Verification items for this drawing (mm, ordinates from the low corner). A direction names the side the tool comes from. Coordinates: 2 decimals unless noted, no trailing zeros. Order: outer loops, then holes, each group sorted by start corner. A loop starts at its lowest first (then second) coordinate and runs counter-clockwise, first axis right, second up. Notation, with made-up numbers: M 52.5,49.5 L 93.5,49.5 A34 cw 93.5,82.5 Z; hole C -22,54 d4. An arc over 180 degrees is marked long. One line per item, written item: value. Start each with the question number.
1) Sectioned sample at D-D, the plane x = 8. Enter the section's corners in (y, z), then the cut area to 3 significant figures.
2) Sectioned sample at C-C, the plane y = 19. Enter the section's corners in (x, z).
3) Access from +Z, -Z, +X, -X, +Y, -Y to the whole of each face (thin tool, end or side, straight path). Record for the marked faces 1, 2 and 3.
4) Go/stop test with flat-tipped pins: P1, Ø2.5, axis at x = 13.5, z = 37, coming from the +Y side; P2, Ø0.9, axis at x = 23, z = 24, coming from the +Y side (1 decimal); P3, Ø0.9, axis at x = 18, z = 35, coming from the +Y side. Record where each tip stops, or that it passes through.
5) Draft check along X on the marked faces 4, 5 and 6. Enter one of: pulls with the +X half, pulls with the -X half, needs draft (parallel to the pull), parting line crosses it, or undercut.
6) Sectioned sample at A-A, the plane y = 29.5. Enter the section's corners in (x, z) (1 decimal).
7) Sectioned sample at B-B, the plane z = 18.5. Enter the section's corners in (x, y) (1 decimal).
8) Thickness scan on L1, parallel to X at y = 4, z = 3 (1 decimal); L2, parallel to X at y = 22, z = 3.5; L3, parallel to X at y = 18, z = 22. Record the ranges inside material, lowest first. Write a range as from..to.
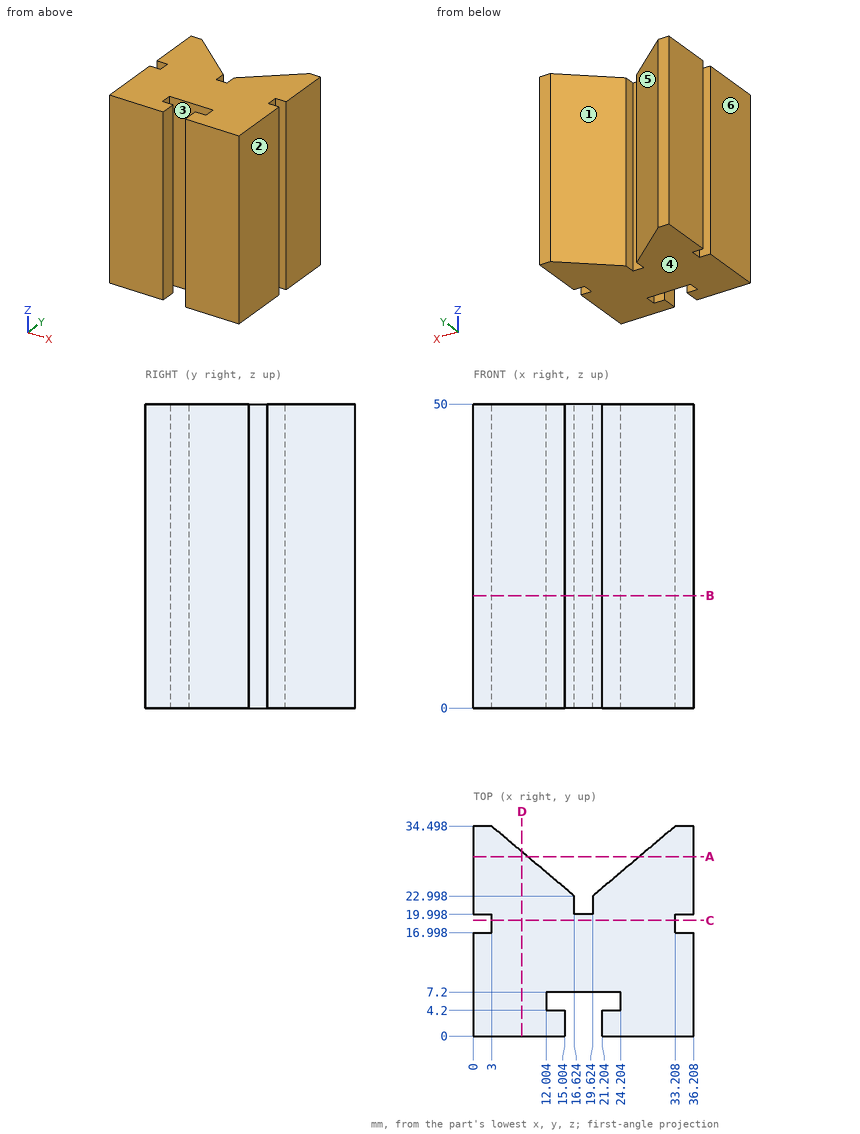
Final values:
1. outline: M 0,0 L 30.28,0 L 30.28,50 L 0,50 Z
1. area: 1,510 mm^2
2. outline: M 3,0 L 33.21,0 L 33.21,50 L 3,50 Z
3. face 1: +Z, -Z, +Y
3. face 2: +Z, -Z, +X, +Y, -Y
3. face 3: +Z, -Z
4. P1: stops at y = 26.69
4. P2: stops at y = 26.2
4. P3: stops at y = 20
5. face 4: needs draft
5. face 5: undercut
5. face 6: pulls with the -X half
6. outline: M 0,0 L 8.9,0 L 8.9,50 L 0,50 Z; M 27.3,0 L 36.2,0 L 36.2,50 L 27.3,50 Z
7. outline: M 0,0 L 15,0 L 15,4.2 L 12,4.2 L 12,7.2 L 24.2,7.2 L 24.2,4.2 L 21.2,4.2 L 21.2,0 L 36.2,0 L 36.2,17 L 33.2,17 L 33.2,20 L 36.2,20 L 36.2,34.5 L 33.2,34.5 L 19.6,23 L 19.6,20 L 16.6,20 L 16.6,23 L 3,34.5 L 0,34.5 L 0,20 L 3,20 L 3,17 L 0,17 Z
8. L1: x = 0..15, 21.2..36.2
8. L2: x = 0..16.62, 19.62..36.21
8. L3: x = 3..33.21
